Geometry check sheet. Reference: the model listing, model coordinates, mm. A direction names the side the tool comes from. Coordinates: 2 decimals unless noted, no trailing zeros. Write each loop counter-clockwise with the first axis right and the second up, starting at its lowest first coordinate (ties: lowest second). Pieces come first, ordered by that corner, then holes. Notation, with made-up numbers: (63.25, 6.25) -> (121.25, 6.25) arc R11 cw to (121.25, 24.25) -> close; hole circle Ø10 at (-27.75, 2.25). An arc over 180 degrees is marked (long way). Put each result on its own line as item: value. Start each with the question number.
Autodesk Fusion 360 part; units mm, degrees
sketch "Sketch1" plane through (0, 0, 0) normal (0, 1, 0) x (1, 0, 0)
  circle A0 centre (0.0008, 24.9355) radius 3
  line L0 (2.5556, 32.9383) -> (-2.4444, 32.9383)
  line L1 (2.5556, 20.6375) -> (2.5556, -15.7025)
  line L2 (8, 25) -> (8, -20)
  circle A1 centre (0, -20) radius 3
  line L3 (-2.6799, 20.7149) -> (-2.6799, -15.7789)
  arc A2 (2.5556, 20.6375) -> (-2.6799, 20.7149) centre (0.0008, 24.9355) ccw
  arc A3 (-2.6799, -15.7789) -> (2.5556, -15.7025) centre (0, -20) ccw
  dimension "d1" = 6
  dimension "d2" = 10
  dimension "d4" = 5
  dimension "d5" = 36.34
  dimension "d6" = 45
  dimension "d7" = 6
sketch "Sketch2" plane through (0, 0, 0) normal (0, 1, 0) x (1, 0, 0)
  circle A0 centre (160, 0) radius 3
  line L0 (165.3043, -12.1067) -> (165.3043, 17.8933)
  line L1 (165.3043, -12.1067) -> (144.0787, -27.9224)
  line L2 (144.0787, -27.9224) -> (124.0787, -27.9224)
  line L3 (124.0787, -27.9224) -> (105.4535, -9.1138)
  line L4 (105.4535, -9.1138) -> (98.3535, -9.1138)
  line L5 (98.3535, -9.1138) -> (98.3535, 10.8862)
  line L6 (98.3535, 10.8862) -> (112.5535, 10.8862)
  line L7 (112.5535, 10.8862) -> (128, 34)
  line L8 (128, 34) -> (153, 34)
  line L9 (153, 34) -> (165.3043, 17.8933)
  circle A1 centre (144.0787, -15.0238) radius 3
  circle A2 centre (124.0787, -15.0238) radius 3
  line L10 (112.4283, -2.9974) -> (127.553, -3)
  line L11 (127.2855, 2.988) -> (112.556, 3)
  arc A3 (127.553, -3) -> (127.2855, 2.988) centre (127.5535, 0) ccw
  arc A4 (112.556, 3) -> (112.6778, -2.9974) centre (112.5535, 0) ccw
  circle A5 centre (128, 28) radius 2
  circle A6 centre (153, 28) radius 2
  dimension "d10" = 6
  dimension "d11" = 30
  dimension "d12" = 26.47
  dimension "d13" = 20
  dimension "d14" = 26.47
  dimension "d15" = 7.1
  dimension "d16" = 20
  dimension "d17" = 14.2
  dimension "d18" = 27.8
  dimension "d19" = 25
  dimension "d21" = 6
  dimension "d22" = 6
  dimension "d23" = 6
  dimension "d24" = 15
  dimension "d25" = 6
  dimension "d26" = 4
  dimension "d27" = 4
sketch "Sketch3" plane through (0, 0, 0) normal (0, 1, 0) x (1, 0, 0)
sketch "Sketch4" plane through (0, 0, 0) normal (0, 1, 0) x (1, 0, 0)
extrude "Extrude2" add sketch "Sketch2" along normal blind 4
sketch "Sketch5" plane through (0, 0, 0) normal (0, 1, 0) x (1, 0, 0)
  circle A0 centre (0, -75) radius 3
  circle A1 centre (-0.0243, -126.973) radius 3
  line L0 (-20, -70) -> (-20, -141.97)
  line L1 (-5, -75) -> (-5, -112.8223)
  line L2 (5, -75) -> (5, -112.8395)
  arc A2 (5, -75) -> (-5, -75) centre (0, -75) ccw
  line L3 (-0.05, -141.973) -> (-0.05, -143.513)
  line L4 (-0.05, -143.513) -> (-0.4621, -143.739)
  line L5 (-0.4621, -143.739) -> (-1.4621, -143.739)
  line L6 (-1.4621, -143.739) -> (-1.9628, -143.2357)
  line L7 (-1.9628, -143.2357) -> (-1.9628, -141.8472)
  line L8 (-0.05, -145.0973) -> (-0.05, -123.9731)
  line L9 (-8.7204, -112.6318) -> (-7.8791, -112.0912)
  line L10 (-8.9448, -113.0448) -> (-8.7204, -112.6318)
  line L11 (-8.1122, -114.3403) -> (-8.9448, -113.0448)
  line L12 (-7.1857, -112.2439) -> (-6.4351, -113.412)
  line L13 (-7.8791, -112.0912) -> (-7.1857, -112.2439)
  line L14 (-12.4085, -115.6627) -> (-11.7536, -114.907)
  line L15 (-12.5075, -116.1222) -> (-12.4085, -115.6627)
  line L16 (-11.3436, -117.1306) -> (-12.5075, -116.1222)
  line L17 (-11.0453, -114.8581) -> (-9.996, -115.7674)
  line L18 (-11.7536, -114.907) -> (-11.0453, -114.8581)
  line L19 (-15.0933, -119.6099) -> (-14.6779, -118.7003)
  line L20 (-15.0589, -120.0786) -> (-15.0933, -119.6099)
  line L21 (-13.658, -120.7184) -> (-15.0589, -120.0786)
  line L22 (-14.012, -118.4539) -> (-12.749, -119.0307)
  line L23 (-14.6779, -118.7003) -> (-14.012, -118.4539)
  line L24 (-16.5573, -124.1536) -> (-16.415, -123.1638)
  line L25 (-16.3922, -124.5936) -> (-16.5573, -124.1536)
  line L26 (-14.8679, -124.8128) -> (-16.3922, -124.5936)
  line L27 (-15.8455, -122.7398) -> (-14.4712, -122.9374)
  line L28 (-16.415, -123.1638) -> (-15.8455, -122.7398)
  line L29 (-16.682, -128.9257) -> (-16.8243, -127.9359)
  line L30 (-16.3995, -129.3014) -> (-16.682, -128.9257)
  line L31 (-14.8752, -129.0822) -> (-16.3995, -129.3014)
  line L32 (-16.3973, -127.3686) -> (-15.023, -127.171)
  line L33 (-16.8243, -127.9359) -> (-16.3973, -127.3686)
  line L34 (-15.4571, -133.5396) -> (-15.8725, -132.63)
  line L35 (-15.0802, -133.8205) -> (-15.4571, -133.5396)
  line L36 (-13.6794, -133.1808) -> (-15.0802, -133.8205)
  line L37 (-15.6226, -131.9654) -> (-14.3596, -131.3886)
  line L38 (-15.8725, -132.63) -> (-15.6226, -131.9654)
  line L39 (-12.9819, -137.6215) -> (-13.6367, -136.8658)
  line L40 (-12.5412, -137.7849) -> (-12.9819, -137.6215)
  line L41 (-11.3773, -136.7764) -> (-12.5412, -137.7849)
  line L42 (-13.5843, -136.1577) -> (-12.5349, -135.2485)
  line L43 (-13.6367, -136.8658) -> (-13.5843, -136.1577)
  line L44 (-9.457, -140.8408) -> (-10.2982, -140.3002)
  line L45 (-8.9881, -140.8734) -> (-9.457, -140.8408)
  line L46 (-8.1555, -139.5779) -> (-8.9881, -140.8734)
  line L47 (-10.4473, -139.606) -> (-9.6967, -138.4379)
  line L48 (-10.2982, -140.3002) -> (-10.4473, -139.606)
  line L49 (-5.1679, -142.9365) -> (-6.1274, -142.6548)
  line L50 (-4.7088, -142.8357) -> (-5.1679, -142.9365)
  line L51 (-4.2749, -141.3581) -> (-4.7088, -142.8357)
  line L52 (-6.466, -142.0308) -> (-6.0748, -140.6985)
  line L53 (-6.1274, -142.6548) -> (-6.466, -142.0308)
  arc A3 (-5, -112.8223) -> (-6.4351, -113.412) centre (-0.0243, -126.973) ccw
  arc A4 (-8.1122, -114.3403) -> (-9.996, -115.7674) centre (-0.0243, -126.973) ccw
  arc A5 (-11.3436, -117.1306) -> (-12.749, -119.0307) centre (-0.0243, -126.973) ccw
  arc A6 (-13.658, -120.7184) -> (-14.4712, -122.9374) centre (-0.0243, -126.973) ccw
  arc A7 (-14.8679, -124.8128) -> (-15.023, -127.171) centre (-0.0243, -126.973) ccw
  arc A8 (-14.8752, -129.0822) -> (-14.3596, -131.3886) centre (-0.0243, -126.973) ccw
  arc A9 (-13.6794, -133.1808) -> (-12.5349, -135.2485) centre (-0.0243, -126.973) ccw
  arc A10 (-11.3773, -136.7764) -> (-9.6967, -138.4379) centre (-0.0243, -126.973) ccw
  arc A11 (-8.1555, -139.5779) -> (-6.0748, -140.6985) centre (-0.0243, -126.973) ccw
  arc A12 (-4.2749, -141.3581) -> (-1.9628, -141.8472) centre (-0.0243, -126.973) ccw
  arc A13 (-0.05, -141.973) -> (5, -112.8395) centre (-0.0243, -126.973) ccw
  dimension "d30" = 6
  dimension "d31" = 10
  dimension "d32" = 6
  dimension "d33" = 30
  dimension "d34" = 71.97
  dimension "d35" = 1.54
  dimension "d36" = 0.47
  dimension "d37" = 1
  dimension "d38" = 0.71
  dimension "d40" = 360
sketch "Sketch6" plane through (0, 0, 0) normal (0, 1, 0) x (1, 0, 0)
  circle A0 centre (135, -70) radius 3
  circle A1 centre (135, -95) radius 3
  line L0 (129.0014, -94.8707) -> (129, -70.0003)
  line L1 (141, -95) -> (141, -70)
  arc A2 (141, -70) -> (129, -70.0003) centre (135, -70) ccw
  line L2 (134.9353, -100.9997) -> (150.363, -126.7288)
  line L3 (138.9186, -99.5437) -> (196.6373, -196.6907)
  arc A3 (129.0014, -94.8707) -> (134.9353, -100.9997) centre (135, -95) ccw
  arc A4 (138.9186, -99.5437) -> (141, -95) centre (135, -95) ccw
  line L4 (196.6373, -196.6907) -> (189.4976, -203.5489)
  line L5 (189.4976, -203.5489) -> (182.5189, -204.0946)
  line L6 (150.363, -126.7288) -> (142.6345, -134.4043)
  line L7 (179.3777, -201.8435) -> (142.738, -137.5509)
  arc A5 (179.3777, -201.8435) -> (182.5189, -204.0946) centre (182.2851, -201.1037) ccw
  arc A6 (142.6345, -134.4043) -> (142.738, -137.5509) centre (145.2387, -135.8936) ccw
  dimension "d43" = 6
  dimension "d44" = 12
  dimension "d45" = 25
  dimension "d46" = 6
  dimension "d47" = 12
  dimension "d48" = 30
  dimension "d50" = 113
  dimension "d52" = 9.9
  dimension "d53" = 7
  dimension "d62" = 6
  dimension "d63" = 74
  dimension "d64" = 6
Item 1: Access from +Z, -Z, +X, -X, +Y, -Y to the whole of each face (thin tool, end or side, straight path). Record for faces 1 (the flat face through (165.304, 2, -3)), 2 (the cylindrical face through (109.554, 1.972, 0.001)), 3 (the flat face through (102, 2, 9.114)).
Item 2: Section check D-D, the plane z = 20. Enter the section's corners in (x, y).
Item 3: Section check A-A, the plane z = 0. Enter the section's corners in (x, y).
Item 4: Mould release check, pull along Z, two halves, no side actions. Record for faces 4 (the cylindrical face through (130.547, 1.972, -0.202)), 5 (the flat face through (120.17, 1.97, -22.28)), 6 (the flat face through (98.354, 2, -1)): released by +Z, released by -Z, zero draft, split by the parting line, or undercut.
Item 5: Section check C-C, the plane y = 0.6. Enter the section's corners in (x, z), and give its area (3 significant figures).
Item 6: Go/stop test with flat-tipped pins: P1, Ø3.5, axis at x = 153, z = -28, coming from the -Y side; P2, Ø2, axis at x = 109.5, y = 0.5, coming from the +Z side; P3, Ø1.2, axis at x = 102, y = 2, coming from the +Z side; P4, Ø1.5, axis at y = 1.5, z = 15.5, coming from the +X side. Record where each tip stops, or that it passes through.
Item 7: Section check B-B, the plane x = 160. Enter the section's corners in (y, z).
Item 8: Scan lines: line 1 along X through (y, z) = (3.1, 0); line 2 along X through (y, z) = (3, -2); line 3 along Z through (x, y) = (126.5, 2.6). Record each from-to range of solid material in increasing order. Write a range as [from, to].
From the geometry:
1. face 1: +Z, -Z, +X, +Y, -Y
1. face 2: +Y, -Y
1. face 3: +Z, -X, +Y, -Y
2. outline: (116.23, 0) -> (154.71, 0) -> (154.71, 4) -> (116.23, 4) -> close
3. outline: (98.35, 0) -> (109.55, 0) -> (109.55, 4) -> (98.35, 4) -> close; (130.55, 0) -> (157, 0) -> (157, 4) -> (130.55, 4) -> close; (163, 0) -> (165.3, 0) -> (165.3, 4) -> (163, 4) -> close
4. face 4: undercut
4. face 5: released by -Z
4. face 6: zero draft
5. outline: (98.35, -10.89) -> (112.55, -10.89) -> (128, -34) -> (153, -34) -> (165.3, -17.89) -> (165.3, 12.11) -> (144.08, 27.92) -> (124.08, 27.92) -> (105.45, 9.11) -> (98.35, 9.11) -> close; hole (112.43, 3) arc R3 ccw to (112.56, -3) -> (127.29, -2.99) arc R3 ccw (long way) to (127.55, 3) -> close; hole circle Ø6 at (124.08, 15.02); hole circle Ø4 at (128, -28); hole circle Ø6 at (144.08, 15.02); hole circle Ø4 at (153, -28); hole circle Ø6 at (160, 0)
5. area: 2,840 mm²
6. P1: through
6. P2: z = 14.21
6. P3: z = 9.11
6. P4: x = 161.76
7. outline: (0, -24.84) -> (4, -24.84) -> (4, -3) -> (0, -3) -> close; (0, 3) -> (4, 3) -> (4, 16.06) -> (0, 16.06) -> close
8. line 1: [98.35, 109.55], [130.55, 157], [163, 165.3]
8. line 2: [98.35, 110.32], [129.79, 157.76], [162.24, 165.3]
8. line 3: [-31.76, -29.32], [-26.68, -2.99], [3, 13.25], [16.8, 27.92]
